Work out the finished part from the listing and answer in its coordinate system (mm). A direction names the side the tool comes from. Coordinates: 2 decimals unless noted, no trailing zeros. Order: outer loops, then holes, each group sorted by start corner. A loop starts at its lowest first (then second) coordinate and runs counter-clockwise, first axis right, second up. Notation, with made-up numbers: (77, 21) -> (82, 21) arc R20 ccw to (82, 40) -> close; hole circle Ø3 at (27.25, 29.5). An arc over 180 degrees is marked (long way). Write item = value, one per line. Start each with the question number.
Q1. Flat-ended cylindrical pins translate along their axes: pin 1 (6 mm diameter, centred on y = 3, z = 5.5, fed in from +X); pin 2 (12 mm diameter, centred on x = 32, y = 14.5, fed in from -Z); pin 3 (3.5 mm diameter, centred on x = 9.5, y = 2, fed in from +Z); pin 4 (3.5 mm diameter, centred on x = 5.5, y = 21, fed in from +Z). Find the tip coordinate at first contact, or state that the pin passes through.
Q2. The part is cut by section C-C, the plane y = 13. Determine the outline of the cut face in (x, z).
Q3. Which of the six approach directions +Z, -Z, +X, -X, +Y, -Y give full straight-line access (tool end or side, diameter ignored) to faces 4 (the cylindrical face through (8.86, 15.43, -6.67)), 5 (the flat face through (28, 14, 5.69)), 6 (the cylindrical face through (23.655, 13.451, 9.239)), 7 (the flat face through (1.224, 9, 10))?
Q4. Straight lines are drawn through the part: L1, parallel to X at y = 16, z = -4.25; L2, parallel to X at y = 16.75, z = 10; L3, parallel to X at y = 23.75, z = 8.75. For each, find the intervals that lie inside material, in ascending order. Write a range as from..to.
Q5. The part is cut by section D-D, the plane x = 27. Determine the outline of the cut face in (y, z), plus the area to 3 significant figures.
Q6. For a pull along X with two mould halves and no side action, classify faces 1 (the cylindrical face through (-7.221, 24.487, 9.239)), 2 (the flat face through (8, 28, 0)), 3 (the flat face through (38.474, 14, 9)) as +X half, -X half, draft (parallel to the pull), parting line (faces both ways), or undercut.
Q7. The part is cut by section A-A, the plane y = 8. Count the separate pieces of the cut face and the enclosed holes in it, plus the area to 3 significant figures.
Q8. The part is cut by section B-B, the plane z = -2. Determine the outline of the cut face in (x, y).
```python
from build123d import *

# Parameters (mm, degrees)
SKETCH1_W                       = 49
SKETCH1_H                       = 25
BOSS_EXTRUDE1_DEPTH             = 28
SKETCH2_W                       = 12.5
SKETCH2_H                       = 5.5
CUT_EXTRUDE1_DEPTH              = 25
F_3_0MM_DOWEL_HOLE1_D           = 3
F_3_0MM_DOWEL_HOLE1_DEPTH       = 11.098709071
F_3_0MM_DOWEL_HOLE1_CSINK_D     = 3.05
F_3_0MM_DOWEL_HOLE1_CSINK_ANGLE = 90
F_3_0MM_DOWEL_HOLE1_TIP         = 0.901290929
F_3_0MM_DOWEL_HOLE2_D           = 3
F_3_0MM_DOWEL_HOLE2_DEPTH       = 24.75
F_3_0MM_DOWEL_HOLE2_CSINK_D     = 3.05
F_3_0MM_DOWEL_HOLE2_CSINK_ANGLE = 90
F_3_0MM_DOWEL_HOLE3_D           = 3
F_3_0MM_DOWEL_HOLE3_CSINK_D     = 3.05
F_3_0MM_DOWEL_HOLE3_CSINK_ANGLE = 90
SKETCH13_R                      = 1.5
CUT_EXTRUDE2_DEPTH              = 12
SKETCH14_W                      = 6.75
SKETCH14_H                      = 18
SKETCH14_W_2                    = 19.75
CUT_EXTRUDE3_DEPTH              = 28
SKETCH15_W                      = 12.5
SKETCH15_H                      = 3
CUT_EXTRUDE4_DEPTH              = 10
CUT_EXTRUDE5_DEPTH              = 11


with BuildPart() as part:
    # Sketch1 → Boss-Extrude1 (new body)
    with BuildSketch(Plane(origin=(0, 0, 0), x_dir=(1, 0, 0), z_dir=(0, 1, 0))):
        with Locations((13.974428044, -0.190405904)):
            Rectangle(SKETCH1_W, SKETCH1_H)
    extrude(amount=BOSS_EXTRUDE1_DEPTH)

    # Sketch2 → Cut-Extrude1 (cut)
    with BuildSketch(Plane(origin=(0, 28, 0), x_dir=(1, 0, 0), z_dir=(0, 1, 0))):
        with Locations((7.474428044, -9.940405904)):
            Rectangle(SKETCH2_W, SKETCH2_H)
    extrude(amount=-CUT_EXTRUDE1_DEPTH, mode=Mode.SUBTRACT)

    # Ø3.0mm Dowel Hole1
    with Locations(Plane(origin=(0, 0, -12.309594096), x_dir=(-1, 0, 0), z_dir=(0, 0, -1))):
        with Locations((-7.474428044, 16)):
            CounterSinkHole(F_3_0MM_DOWEL_HOLE1_D / 2, F_3_0MM_DOWEL_HOLE1_CSINK_D / 2, depth=F_3_0MM_DOWEL_HOLE1_DEPTH, counter_sink_angle=F_3_0MM_DOWEL_HOLE1_CSINK_ANGLE)
            with Locations((0, 0, -(F_3_0MM_DOWEL_HOLE1_DEPTH + F_3_0MM_DOWEL_HOLE1_TIP / 2))):  # 118° drill point
                Cone(0, F_3_0MM_DOWEL_HOLE1_D / 2, F_3_0MM_DOWEL_HOLE1_TIP, mode=Mode.SUBTRACT)

    # Ø3.0mm Dowel Hole2
    with Locations(Plane(origin=(38.474428044, 0, 0), x_dir=(0, 0, -1), z_dir=(1, 0, 0))):
        with Locations((-9.190405904, 8)):
            CounterSinkHole(F_3_0MM_DOWEL_HOLE2_D / 2, F_3_0MM_DOWEL_HOLE2_CSINK_D / 2, depth=F_3_0MM_DOWEL_HOLE2_DEPTH, counter_sink_angle=F_3_0MM_DOWEL_HOLE2_CSINK_ANGLE)

    # Ø3.0mm Dowel Hole3 (through all)
    with Locations(Plane(origin=(0, 0, 0), x_dir=(-1, 0, 0), z_dir=(0, -1, 0))):
        with Locations((-7.474428044, -3.690405904)):
            CounterSinkHole(F_3_0MM_DOWEL_HOLE3_D / 2, F_3_0MM_DOWEL_HOLE3_CSINK_D / 2, counter_sink_angle=F_3_0MM_DOWEL_HOLE3_CSINK_ANGLE)

    # Sketch13 → Cut-Extrude2 (cut)
    with BuildSketch(Plane.XY.offset(12.690405904)):
        with Locations((-7.025571956, 23)):
            Circle(SKETCH13_R)
        with Locations((-7.025571956, 13)):
            Circle(SKETCH13_R)
        with Locations((22.224428044, 23)):
            Circle(SKETCH13_R)
        with Locations((22.224428044, 13)):
            Circle(SKETCH13_R)
    extrude(amount=-CUT_EXTRUDE2_DEPTH, mode=Mode.SUBTRACT)

    # Sketch14 → Cut-Extrude3 (cut)
    with BuildSketch(Plane(origin=(0, 28, 0), x_dir=(1, 0, 0), z_dir=(0, 1, 0))):
        with Locations((-7.150571956, 3.309594096)):
            Rectangle(SKETCH14_W, SKETCH14_H)
        with Locations((28.599428044, 3.309594096)):
            Rectangle(SKETCH14_W_2, SKETCH14_H)
    extrude(amount=-CUT_EXTRUDE3_DEPTH, mode=Mode.SUBTRACT)

    # Sketch15 → Cut-Extrude4 (cut)
    with BuildSketch(Plane(origin=(0, 3, 0), x_dir=(1, 0, 0), z_dir=(0, 1, 0))):
        with Locations((7.474428044, -11.190405904)):
            Rectangle(SKETCH15_W, SKETCH15_H)
    extrude(amount=-CUT_EXTRUDE4_DEPTH, mode=Mode.SUBTRACT)

    # Sketch16 → Cut-Extrude5 (cut)
    with BuildSketch(Plane(origin=(0, 28, 0), x_dir=(1, 0, 0), z_dir=(0, 1, 0))):
        Polygon((14.224428044, -12.690405904), (14.224428044, -6.690405904), (0.724428044, -6.690405904), (0.724428044, -12.690405904), (1.224428044, -12.690405904), (1.224428044, -7.190405904), (13.724428044, -7.190405904), (13.724428044, -12.690405904), align=None)
    extrude(amount=-CUT_EXTRUDE5_DEPTH, mode=Mode.SUBTRACT)


solid = part.part
```
Model answer:
q1.pin_1 = 38.47
q1.pin_2 = 5.69
q1.pin_3 = 9.69
q1.pin_4 = 6.69
q2.outline = (-10.53, 5.69) -> (-8.53, 5.69) -> (-8.53, 12.69) -> (-10.53, 12.69) -> close; (-5.53, 5.69) -> (-3.78, 5.69) -> (-3.78, -12.31) -> (18.72, -12.31) -> (18.72, 5.69) -> (20.72, 5.69) -> (20.72, 12.69) -> (13.72, 12.69) -> (13.72, 7.19) -> (1.22, 7.19) -> (1.22, 12.69) -> (-5.53, 12.69) -> close; (23.72, 5.69) -> (38.47, 5.69) -> (38.47, 12.69) -> (23.72, 12.69) -> close; hole circle Ø3 at (7.47, 3.69)
q3.face_4 = -Z
q3.face_5 = -Z, +X, +Y, -Y
q3.face_6 = +Z, -Z
q3.face_7 = +Z, +Y
q4.L1 = -3.78..5.97, 8.97..18.72
q4.L2 = -10.53..1.22, 13.72..38.47
q4.L3 = -10.53..-8.32, -5.73..0.72, 14.22..20.93, 23.52..38.47
q5.outline = (0, 5.69) -> (28, 5.69) -> (28, 12.69) -> (0, 12.69) -> close; hole circle Ø3 at (8, 9.19)
q5.area = 189 mm2
q6.face_1 = undercut
q6.face_2 = draft
q6.face_3 = +X half
q7.separate_pieces = 2
q7.enclosed_holes = 1
q7.area = 598 mm2
q8.outline = (-3.78, 0) -> (18.72, 0) -> (18.72, 28) -> (-3.78, 28) -> close; hole circle Ø3 at (7.47, 16)
